Autodesk Inventor part; units mm, degrees
ref_plane "YZ Plane" through (0, 0, 0) normal (1, 0, 0) x (0, 1, 0)
ref_plane "XZ Plane" through (0, 0, 0) normal (0, 1, 0) x (-1, 0, 0)
ref_plane "XY Plane" through (0, 0, 0) normal (0, 0, 1) x (1, 0, 0)
sketch "Skizze1" plane through (0, 0, 0) normal (0, 0, 1) x (1, 0, 0)
  line L0 (19.1421, 31.2132) -> (19.1421, 61.2132)
  line L1 (19.1421, 61.2132) -> (39.9308, 61.2132)
  line L2 (39.9308, 61.2132) -> (39.9308, 31.2132)
  line L3 (39.9308, 31.2132) -> (37.9308, 31.2132)
  line L4 (37.9308, 31.2132) -> (37.9308, 26.2132)
  line L5 (37.9308, 26.2132) -> (39.9308, 26.2132)
  line L6 (39.9308, 26.2132) -> (39.9308, 11.2132)
  line L7 (19.1421, 31.2132) -> (21.1421, 31.2132)
  line L8 (21.1421, 31.2132) -> (21.1421, 26.2132)
  line L9 (21.1421, 26.2132) -> (19.1421, 26.2132)
  line L10 (19.1421, 26.2132) -> (19.1421, 11.2132)
  line L11 (39.9308, 41.2132) -> (44.9308, 41.2132)
  line L12 (44.9308, 41.2132) -> (44.9308, 21.2132)
  line L13 (19.1421, 41.2132) -> (14.1421, 41.2132)
  line L14 (14.1421, 41.2132) -> (14.1421, 21.2132)
  line L15 (14.1421, 21.2132) -> (-3.5355, 3.5355)
  arc A0 (-3.5355, 3.5355) -> (-3.2818, -3.7722) centre (0, 0) ccw
  line L16 (44.9308, 21.2132) -> (62.6085, 3.5355)
  arc A1 (62.3548, -3.7722) -> (62.6085, 3.5355) centre (59.073, 0) ccw
  arc A2 (-3.2818, -3.7722) -> (62.3548, -3.7722) centre (29.5365, 33.9499) ccw
  arc A3 (19.1421, 11.2132) -> (39.9308, 11.2132) centre (29.5365, 33.9499) ccw
  line L17 (29.5365, 33.9499) -> (29.5365, 10.2757) construction
  dimension "d0" = 90
  dimension "d1" = 5
  dimension "d2" = 50
  dimension "d3" = 25
  dimension "d4" = 20
  dimension "d5" = 10
  dimension "d6" = 5
  dimension "d7" = 5
  dimension "d8" = 30
  dimension "d9" = 2
  dimension "d10" = 15
  dimension "d11" = 25
extrude "Extrusion1" add sketch "Skizze1" along normal mid plane 10 contours L0 L1 L2 L3 L4 L5 L6 A3 L10 L9 L8 L7
extrude "Extrusion2" add sketch "Skizze1" along normal mid plane 20 contours L7 L8 L9 L10 A3 L6 L5 L4 L3 L2 L11 L12 L16 A1 A2 A0 L15 L14 L13 L0
sketch "Skizze2" plane through (0, 0, 5) normal (0, 0, 1) x (1, 0, 0)
  line L0 (39.9308, 61.2132) -> (19.1421, 61.2132)
  line L1 (29.5365, 61.2132) -> (29.5365, 18.1861) construction
  point P0 (0, 0)
  point P1 (29.5365, 46.2132)
  dimension "d16" = 15
hole "Bohrung1" at (29.5365, 46.2132, 5) direction (0, 0, -1) diameter 10 depth 10
chamfer "Fasen1" distance 1 angle 45 2 edges at (29.5365, 8.9499, 10) (29.5365, 8.9499, -10)
sketch "Skizze3" plane through (0, 0, 10) normal (0, 0, 1) x (1, 0, 0)
  arc A0 (6.4055, -2.2397) -> (53.6752, -1.5754) centre (29.5365, 33.9499) ccw construction
  arc A1 (-3.2818, -3.7722) -> (62.3548, -3.7722) centre (29.5365, 33.9499) ccw
  point P0 (0, 0)
  point P1 (21.3005, -8.2034)
  point P2 (31.2715, -8.9654)
  point P3 (41.2715, -7.3662)
  point P4 (51.2715, -3.0949)
  point P5 (11.3005, -4.9369)
  dimension "d27" = 10
  dimension "d28" = 10
  dimension "d29" = 10
  dimension "d30" = 10
hole "Bohrung2" at (21.3005, -8.2034, 10) at (31.2715, -8.9654, 10) at (41.2715, -7.3662, 10) at (51.2715, -3.0949, 10) at (11.3005, -4.9369, 10) direction (0, 0, -1) diameter 6 end through all
fillet "Rundung1" radius 2 2 edges at (19.1421, 61.2132, 0) (39.9308, 61.2132, 0)
properties part number "werkzeug" material "Stahl, galvanisiert"
Verification items for the finished model (mm, model axes). A direction names the side the tool comes from. Coordinates: 2 decimals unless noted, no trailing zeros. Write each loop counter-clockwise with the first axis right and the second up, starting at its lowest first coordinate (ties: lowest second). Pieces come first, ordered by that corner, then holes. Notation, with made-up numbers: (-9, 41) - (14, 41) arc R17 cw to (14, 67) - close; hole circle Ø2 at (39, 19). An arc over 180 degrees is marked (long way). Answer as a JSON object with one key per item and string values.
(1) Gauge pin test, flat ends, axial feed: pin 1 Ø1.6 at (x, z) = (39, -8) entering from +Y; pin 2 Ø6 at (x, z) = (42.5, 5.5) entering from +Y; pin 3 Ø4 at (x, z) = (46.5, -0.5) entering from -Y; pin 4 Ø2 at (x, y) = (21, 10) entering from +Z. Record the tip position at first contact, or that the pin passes through.
Report:
{"pin 1": "y = 31.21", "pin 2": "y = 60.4", "pin 3": "y = -13.76", "pin 4": "z = 10"}
(2) Cross-section at D-D on x = 53. Record the cut outline in (y, z).
Report:
{"outline": "(-10.2, -10) - (-5.55, -10) - (-5.55, 10) - (-10.2, 10) - close; (-0.64, -10) - (13.14, -10) - (13.14, 10) - (-0.64, 10) - close"}
(3) Cross-section at A-A on y = 23. Record the cut outline in (x, z).
Report:
{"outline": "(14.14, -10) - (19.14, -10) - (19.14, -5) - (39.93, -5) - (39.93, -10) - (44.93, -10) - (44.93, 10) - (39.93, 10) - (39.93, 5) - (19.14, 5) - (19.14, 10) - (14.14, 10) - close"}
(4) Cross-section at B-B on z = -7. Record the cut outline in (x, y), plus the area to 3 significant figures.
Report:
{"outline": "(-3.54, 3.54) arc R5 ccw to (-3.28, -3.77) arc R50 ccw to (62.35, -3.77) arc R5 ccw to (62.61, 3.54) - (44.93, 21.21) - (44.93, 41.21) - (39.93, 41.21) - (39.93, 31.21) - (37.93, 31.21) - (37.93, 26.21) - (39.93, 26.21) - (39.93, 11.21) arc R25 cw to (19.14, 11.21) - (19.14, 26.21) - (21.14, 26.21) - (21.14, 31.21) - (19.14, 31.21) - (19.14, 41.21) - (14.14, 41.21) - (14.14, 21.21) - close; hole circle Ø6 at (11.3, -4.94); hole circle Ø6 at (21.3, -8.2); hole circle Ø6 at (31.27, -8.97); hole circle Ø6 at (41.27, -7.37); hole circle Ø6 at (51.27, -3.09)", "area": "1,750 mm^2"}
(5) Tool access check on faces 5 (the flat face through (19.142, 18, -8)), 6 (the flat face through (44.931, 31, 0)), 7 (the cylindrical face through (29.69, 8.95, 6.97)), 8 (the flat face through (19.142, 36, -8)). Record the directions out of +Z, -Z, +X, -X, +Y, -Y that give a thin tool (end or side, any length) a straight path to the whole face; none if there is none.
Report:
{"face 5": "-Z", "face 6": "+Z, -Z, +X, +Y", "face 7": "+Z", "face 8": "-Z, +Y"}
(6) Cross-section at C-C on y = 45. Record the cut outline in (x, z).
Report:
{"outline": "(19.14, -5) - (24.69, -5) - (24.69, 5) - (19.14, 5) - close; (34.39, -5) - (39.93, -5) - (39.93, 5) - (34.39, 5) - close"}
(7) Mould release check, pull along Y, two halves, no side actions. Record for faces 1 (the flat face through (39, 31.213, 7)), 2 (the cylindrical face through (-5, 0, 0)), 3 (the flat face through (29, 7, -10)), 4 (the cylindrical face through (20.399, -11.065, -0.14)): pulls with the +Y half, pulls with the -Y half, needs draft (parallel to the pull), parting line crosses it, or undercut.
Report:
{"face 1": "pulls with the +Y half", "face 2": "parting line crosses it", "face 3": "needs draft", "face 4": "undercut"}
(8) Thickness scan on line 1 along X through (y, z) = (-8, 4); line 2 along Z through (x, y) = (35, 18); line 3 along Y through (x, z) = (10.5, -1.75). Record the ranges inside material, lowest first.
Report:
{"line 1": "2.33 to 18.31, 24.29 to 28.43, 34.11 to 38.34, 44.2 to 56.74", "line 2": "-5 to 5", "line 3": "-12.28 to -7.83, -2.05 to 17.57"}
